Design review of the part built by this model. Coordinates are the model's own, in mm. Coordinates: 2 decimals unless noted, no trailing zeros. Loops run counter-clockwise (first coordinate to the right, second up) from the corner with the lowest first, then second, coordinate; pieces in that order, holes last.
Q1. Add section A-A on x = 41. Give the boundary of the cut face in (y, z), and give its area (3 significant figures).
Q2. For P1, Ø4.5, axis at x = 169.89, y = -3.58, coming from the -Z side; P2, Ø2.5, axis at x = 156.81, y = 38.66, coming from the +Z side; P3, Ø1.5, axis at x = -33, z = 3, coming from the -Y side; P4, Ø2, axis at x = 96, z = 1.5, coming from the +Y side, all flat-tipped, find the tip position at first contact; note any pin that passes through.
Q3. Wall thickness on probe 1 along X at (y, z) = (-156, 2); probe 2 along X at (y, z) = (29.5, 1); probe 3 along Y at (x, z) = (142, 2.5): over which ranges is each line inside the solid? List them lowest first.
Q4. Add section B-B on z = 1. Give the number of separate pieces and of enclosed holes in the cut face, and give its area (3 significant figures).
```python
from build123d import *

# Parameters (mm, degrees)
SKETCH1_W           = 63.5
SKETCH1_H           = 6.35
BOSS_EXTRUDE1_DEPTH = 6.35
SKETCH7_R           = 1.4224
SKETCH7_R_2         = 1.63195
CUT_EXTRUDE4_DEPTH  = 257.697479146
SKETCH3_R           = 1.4605
CUT_EXTRUDE5_DEPTH  = 257.697479146
CUT_EXTRUDE6_DEPTH  = 257.697479146
SKETCH10_R          = 1.4224
CUT_EXTRUDE7_DEPTH  = 257.697479146
SKETCH11_R          = 1.4224
CUT_EXTRUDE8_DEPTH  = 257.697479146


with BuildPart() as part:
    # Sketch1 → Boss-Extrude1 (new body)
    with BuildSketch(Plane.XY):
        Polygon((-1.941106456, 35.484446355), (-65.441106456, 35.484446355), (-65.441106456, -167.715553645), (-1.941106456, -167.715553645), (61.558893544, -167.715553645), (61.558893544, -174.065553645), (125.058893544, -174.065553645), (125.058893544, -167.715553645), (188.558893544, -167.715553645), (188.558893544, 41.834446355), (125.058893544, 41.834446355), (125.058893544, 35.484446355), align=None)
        with Locations((-33.691106456, 38.659446355)):
            Rectangle(SKETCH1_W, SKETCH1_H)
        with Locations((29.808893544, -170.890553645)):
            Rectangle(SKETCH1_W, SKETCH1_H)
    extrude(amount=BOSS_EXTRUDE1_DEPTH)

    # Sketch7 → Cut-Extrude4 (cut, through all)
    with BuildSketch(Plane.XY.offset(6.35)):
        with Locations((108.548893544, 18.974446355)):
            Circle(SKETCH7_R)
        with Locations((83.148893544, 18.974446355)):
            Circle(SKETCH7_R)
        with Locations((92.546893544, -27.837753645)):
            Circle(SKETCH7_R_2)
        with Locations((114.771644595, -27.942947347)):
            Circle(SKETCH7_R_2)
        with Locations((67.908893544, -88.975553645)):
            Circle(SKETCH7_R)
        with Locations((98.388893544, -88.975553645)):
            Circle(SKETCH7_R)
        with Locations((98.388893544, -110.565553645)):
            Circle(SKETCH7_R)
        with Locations((67.908893544, -110.565553645)):
            Circle(SKETCH7_R)
        with Locations((141.568893544, -151.205553645)):
            Circle(SKETCH7_R)
        with Locations((166.968893544, -151.205553645)):
            Circle(SKETCH7_R)
        with Locations((135.346142493, -104.288159943)):
            Circle(SKETCH7_R_2)
        with Locations((157.570893544, -104.393353645)):
            Circle(SKETCH7_R_2)
        with Locations((151.728893544, -43.255553645)):
            Circle(SKETCH7_R)
        with Locations((151.728893544, -21.665553645)):
            Circle(SKETCH7_R)
        with Locations((182.208893544, -43.255553645)):
            Circle(SKETCH7_R)
        with Locations((182.208893544, -21.665553645)):
            Circle(SKETCH7_R)
    extrude(amount=-CUT_EXTRUDE4_DEPTH, mode=Mode.SUBTRACT)

    # Sketch3 → Cut-Extrude5 (cut, through all)
    with BuildSketch(Plane.XY.offset(6.35)):
        with Locations((156.808893544, 38.659446355)):
            Circle(SKETCH3_R)
        with Locations((29.808893544, -170.890553645)):
            Circle(SKETCH3_R)
        with Locations(Location((93.308893544, -170.890553645, 0), (0, 0, 180))):
            Circle(SKETCH3_R)
        with Locations(Location((-33.691106456, 38.659446355, 0), (0, 0, 180))):
            Circle(SKETCH3_R)
    extrude(amount=-CUT_EXTRUDE5_DEPTH, mode=Mode.SUBTRACT)

    # Sketch8 → Cut-Extrude6 (cut, through all)
    with BuildSketch(Plane(origin=(0, 0, 0), x_dir=(-1, 0, 0), z_dir=(0, 0, -1))):
        Polygon((-91.784893544, 35.484446355), (-94.832893544, 35.484446355), (-94.832893544, 31.674446355), (-96.610893544, 31.674446355), (-96.610893544, 29.134446355), (-94.832893544, 29.134446355), (-94.832893544, 22.784446355), (-91.784893544, 22.784446355), (-91.784893544, 29.134446355), (-90.006893544, 29.134446355), (-90.006893544, 31.674446355), (-91.784893544, 31.674446355), align=None)
        Polygon((-155.284893544, -167.715553645), (-158.332893544, -167.715553645), (-158.332893544, -163.905553645), (-160.110893544, -163.905553645), (-160.110893544, -161.365553645), (-158.332893544, -161.365553645), (-158.332893544, -155.015553645), (-155.284893544, -155.015553645), (-155.284893544, -161.365553645), (-153.506893544, -161.365553645), (-153.506893544, -163.905553645), (-155.284893544, -163.905553645), align=None)
        Polygon((-31.332893544, 35.484446355), (-28.284893544, 35.484446355), (-28.284893544, 31.674446355), (-26.506893544, 31.674446355), (-26.506893544, 29.134446355), (-28.284893544, 29.134446355), (-28.284893544, 22.784446355), (-31.332893544, 22.784446355), (-31.332893544, 29.134446355), (-33.110893544, 29.134446355), (-33.110893544, 31.674446355), (-31.332893544, 31.674446355), align=None)
        Polygon((32.167106456, -167.715553645), (32.167106456, -163.905553645), (30.389106456, -163.905553645), (30.389106456, -161.365553645), (32.167106456, -161.365553645), (32.167106456, -155.015553645), (35.215106456, -155.015553645), (35.215106456, -161.365553645), (36.993106456, -161.365553645), (36.993106456, -163.905553645), (35.215106456, -163.905553645), (35.215106456, -167.715553645), align=None)
    extrude(amount=-CUT_EXTRUDE6_DEPTH, mode=Mode.SUBTRACT)

    # Sketch10 → Cut-Extrude7 (cut, through all)
    with BuildSketch(Plane.XY.offset(6.35)):
        with Locations((169.889893544, -3.575553701)):
            Circle(SKETCH10_R)
        with Locations((169.889893544, 23.094446299)):
            Circle(SKETCH10_R)
        with Locations((147.664893544, -11.830553701)):
            Circle(SKETCH10_R)
    extrude(amount=-CUT_EXTRUDE7_DEPTH, mode=Mode.SUBTRACT)

    # Sketch11 → Cut-Extrude8 (cut, through all)
    with BuildSketch(Plane.XY.offset(6.35)):
        with Locations((-25.428800612, -7.905553469)):
            Circle(SKETCH11_R)
        with Locations((-25.428800612, -34.575553469)):
            Circle(SKETCH11_R)
        with Locations((35.531199388, -34.575553469)):
            Circle(SKETCH11_R)
        with Locations((35.531199388, -7.905553469)):
            Circle(SKETCH11_R)
    extrude(amount=-CUT_EXTRUDE8_DEPTH, mode=Mode.SUBTRACT)


solid = part.part
```
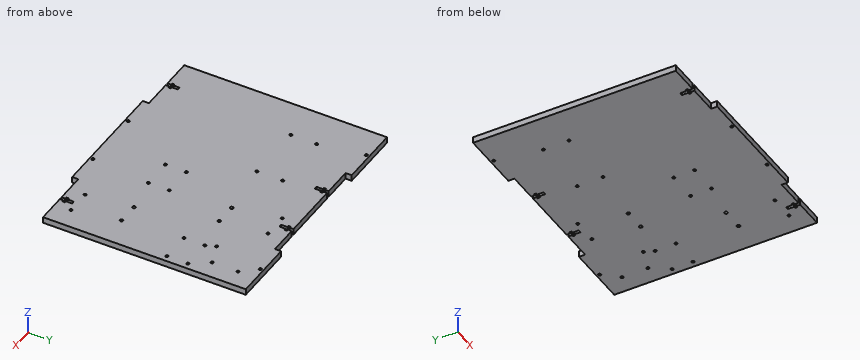
Entries:
1. outline: (-174.07, 0) - (35.48, 0) - (35.48, 6.35) - (-174.07, 6.35) - close
1. area: 1,330 mm2
2. P1: stops at z = 0
2. P2: passes through
2. P3: stops at y = -155.02
2. P4: stops at y = 35.48
3. probe 1: x = -65.44 to -35.22, -32.17 to 155.28, 158.33 to 188.56
3. probe 2: x = -65.44 to 26.51, 33.11 to 90.01, 96.61 to 188.56
3. probe 3: y = -167.72 to -152.56, -149.85 to 41.83
4. separate pieces: 1
4. enclosed holes: 27
4. area: 52,900 mm2
